Can you work these out from the drawing? Everything is in mm from the part's minimum corner. Give positions to 0.01 mm unless a question says otherwise; leave off trailing zeros. Loops run counter-clockwise (first coordinate to the right, second up) from the corner with the lowest first, then second, coordinate; pieces in that order, holes last. Notation, with made-up numbers: (28.25, 47) - (41.25, 47) arc R16 cw to (41.25, 72) - close; hole circle Ø6 at (-24.75, -13.75). An arc over 180 degrees is marked (long way). Answer in a Markdown table with one row per item.
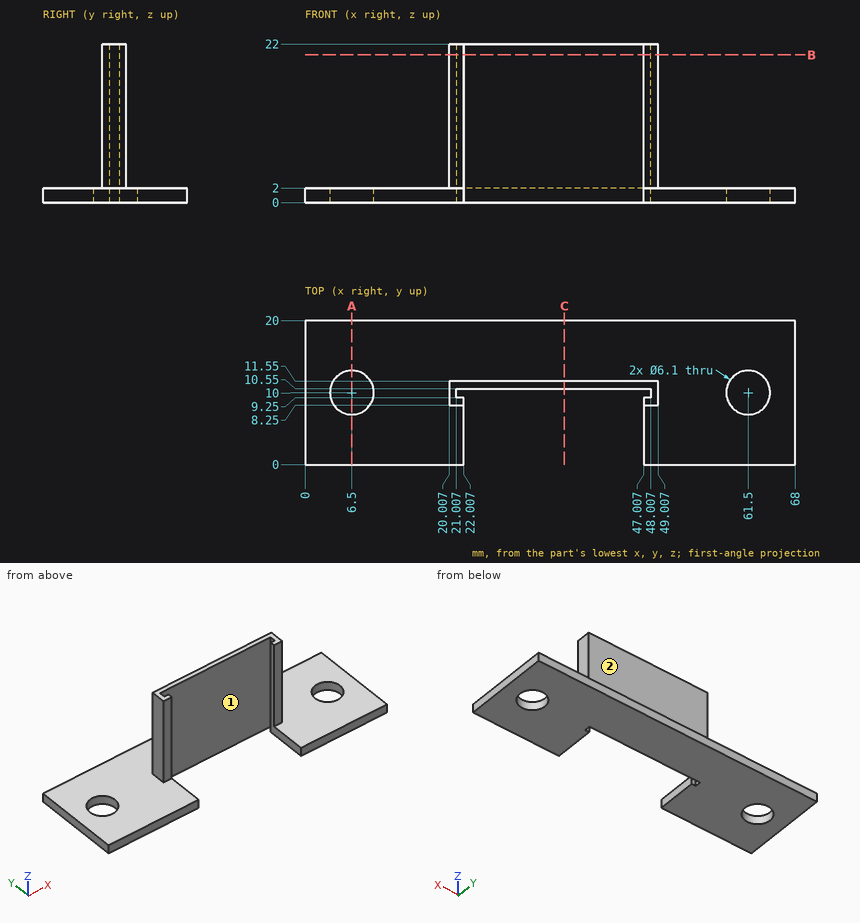
Q1. Imagine slicing it at A-A, the plane x = 6.5. Write out the boundary of the cut face in (y, z).
Checked values:
| item | result |
|---|---|
| outline | (0, 0) - (6.95, 0) - (6.95, 2) - (0, 2) - close; (13.05, 0) - (20, 0) - (20, 2) - (13.05, 2) - close |
Q2. Imagine slicing it at C-C, the plane x = 36. Write out the boundary of the cut face in (y, z), and give its area (3 significant figures).
Checked values:
| item | result |
|---|---|
| outline | (10.55, 0) - (20, 0) - (20, 2) - (11.55, 2) - (11.55, 22) - (10.55, 22) - close |
| area | 38.9 mm² |
Q3. If we mould it in two halves opening along X, with no side actions, what happens to the marked faces 1 and 2? For each: released by +X, released by -X, zero draft, split by the parting line, or undercut.
Checked values:
| item | result |
|---|---|
| face 1 | undercut |
| face 2 | zero draft |
Q4. If I drill on line 1 (X direction, y = 8.75, z = 5.5); line 2 (Y direction, x = 6.5, z = 0.8); line 3 (X direction, y = 11, z = 1.25), over which ranges is the centre line in solid material (lowest first)? Write a range as [from, to].
Checked values:
| item | result |
|---|---|
| line 1 | x = [20.01, 22.01], [47.01, 49.01] |
| line 2 | y = [0, 6.95], [13.05, 20] |
| line 3 | x = [0, 3.62], [9.38, 58.62], [64.38, 68] |
Q5. Imagine slicing it at B-B, the plane z = 20.5. Write out the boundary of the cut face in (x, y).
Checked values:
| item | result |
|---|---|
| outline | (20.01, 8.25) - (22.01, 8.25) - (22.01, 9.25) - (21.01, 9.25) - (21.01, 10.55) - (48.01, 10.55) - (48.01, 9.25) - (47.01, 9.25) - (47.01, 8.25) - (49.01, 8.25) - (49.01, 11.55) - (20.01, 11.55) - close |
Q6. For pin 1 (1 mm diameter, centred on y = 10, z = 7, fed in from -X); pin 2 (3.5 mm diameter, centred on x = 6.5, y = 10, fed in from -Z); pin 3 (1.1 mm diameter, centred on x = 21.5, z = 9, fed in from +Y); pin 4 (1 mm diameter, centred on x = 21.5, z = 7, fed in from -Y), each with a flat end and sliding along its axis, tell me the tip position at first contact or that it passes through.
Checked values:
| item | result |
|---|---|
| pin 1 | stops at x = 20.01 |
| pin 2 | passes through |
| pin 3 | stops at y = 11.55 |
| pin 4 | stops at y = 8.25 |
